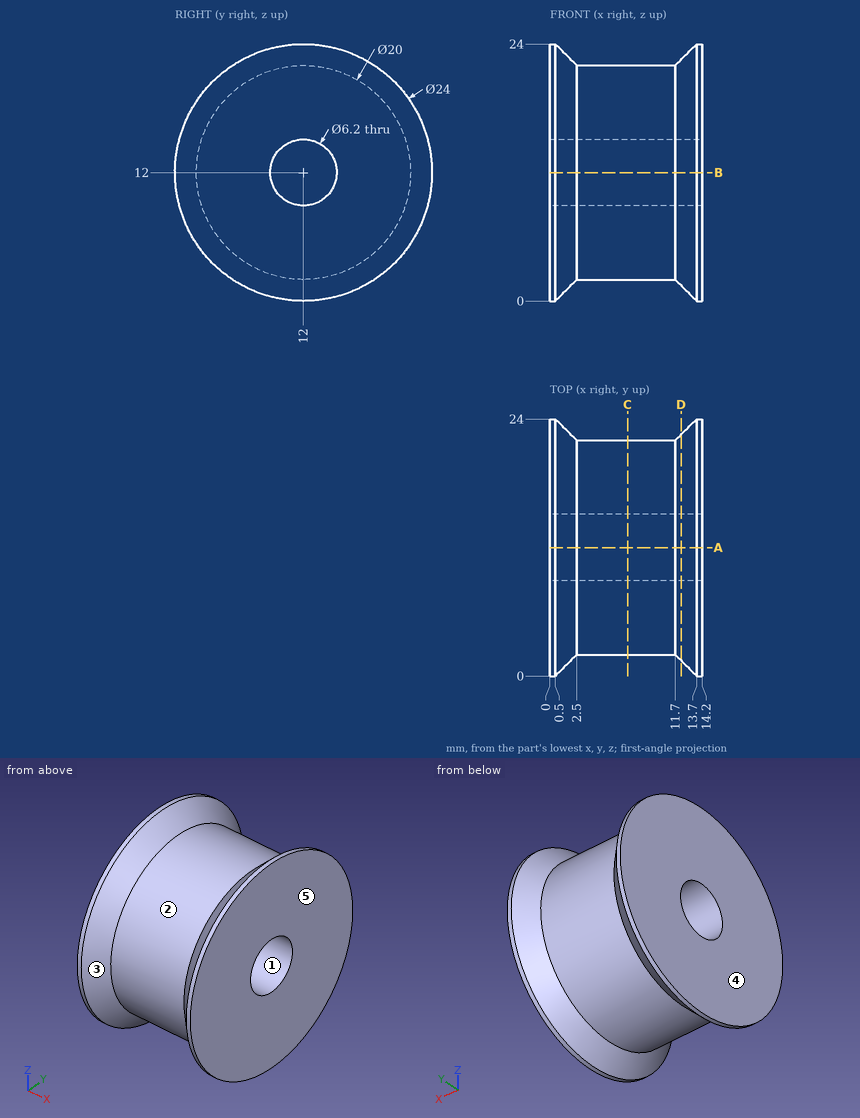
Source: three-view drawing plus pictorial views. Frame: mm from the lowest corner of the part. A direction names the side the tool comes from. Coordinates: 2 decimals unless noted, no trailing zeros. Order: outer loops, then holes, each group sorted by start corner. A loop starts at its lowest first (then second) coordinate and runs counter-clockwise, first axis right, second up.
1) Ray query, probe 1 along Y at (x, z) = (3.25, 12); probe 2 along Z at (x, y) = (11.5, 13.5); probe 3 along X at (y, z) = (14, 1.75). Return the intervals inside material, ascending.
Result sheet:
probe 1: y = 2 to 8.9, 15.1 to 22
probe 2: z = 2.11 to 9.29, 14.71 to 21.89
probe 3: x = 0 to 2.06, 12.14 to 14.2
2) Draft query along X for the marked faces 3, 4 and 5. Return one class per face: released by +X, released by -X, zero draft, split by the parting line, or undercut.
Result sheet:
face 3: undercut
face 4: released by -X
face 5: released by +X
3) Section D-D (x = 12.25). Return loops of the section in (y, z).
Result sheet:
outline: circle Ø21.1 at (12, 12); hole circle Ø6.2 at (12, 12)
4) First-contact query: P1, Ø4, axis at x = 6, y = 3, coming from the -Z side; P2, Ø2, axis at x = 6.5, z = 12, coming from the -Y side; P3, Ø1.5, axis at x = 5, y = 11.5, coming from the -Z side; P4, Ø5.5, axis at y = 12, z = 12, coming from the +X side. Flat tips, straight axial feed; report the tip coordinate or a pass-through.
Result sheet:
P1: stops at z = 4.86
P2: stops at y = 2
P3: stops at z = 2
P4: passes through
5) Section C-C (x = 7.25). Return loops of the section in (y, z), then the cut area to 3 significant figures.
Result sheet:
outline: circle Ø20 at (12, 12); hole circle Ø6.2 at (12, 12)
area: 284 mm2
6) Section A-A (y = 12). Return loops of the section in (x, z), then the cut area to 3 significant figures.
Result sheet:
outline: (0, 0) - (0.5, 0) - (2.5, 2) - (11.7, 2) - (13.7, 0) - (14.2, 0) - (14.2, 8.9) - (0, 8.9) - close; (0, 15.1) - (14.2, 15.1) - (14.2, 24) - (13.7, 24) - (11.7, 22) - (2.5, 22) - (0.5, 24) - (0, 24) - close
area: 208 mm2
7) Set-up query: the marked faces 1 and 2. Return all of +Z, -Z, +X, -X, +Y, -Y with unobstructed straight access to the full face (end or side cutting, diameter ignored); none if empty.
Result sheet:
face 1: +X, -X
face 2: none
